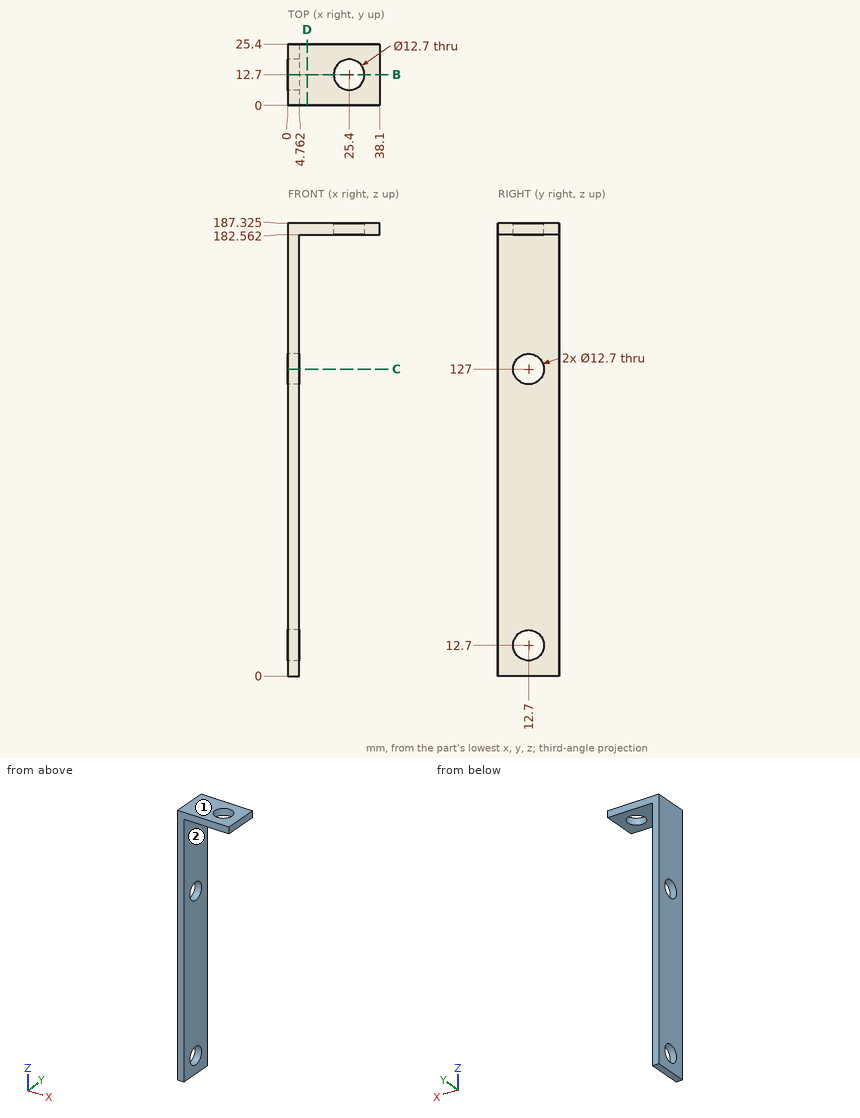
Source: three-view drawing plus pictorial views. Frame: mm from the lowest corner of the part. A direction names the side the tool comes from. Give positions to 0.01 mm unless a question says otherwise; leave off trailing zeros. Order: outer loops, then holes, each group sorted by start corner. A loop starts at its lowest first (then second) coordinate and runs counter-clockwise, first axis right, second up. Notation, with made-up numbers: (13, 35.25) -> (36, 35.25) arc R19 cw to (36, 63.25) -> close; hole circle Ø7 at (-20, 67.5). An arc over 180 degrees is marked (long way). Use a Markdown table: item, result.
Q1. Section C-C (z = 127). Return the cut outline in (x, y).
A:
| item | result |
|---|---|
| outline | (0, 0) -> (4.76, 0) -> (4.76, 6.35) -> (0, 6.35) -> close; (0, 19.05) -> (4.76, 19.05) -> (4.76, 25.4) -> (0, 25.4) -> close |
Q2. Material intervals for line 1 (Y direction, x = 25.4, z = 185.4); line 2 (X direction, y = 5, z = 92); line 3 (Z direction, x = 17, y = 13) (1 decimal), sorted ascending. Write a range as [from, to].
A:
| item | result |
|---|---|
| line 1 | [0, 6.35], [19.05, 25.4] |
| line 2 | [0, 4.76] |
| line 3 | [182.6, 187.3] |
Q3. Access query for the marked faces 1 and 2. Directions: +Z, -Z, +X, -X, +Y, -Y. A direction counts if a zero-diameter tool reaches every point of the face in a straight line with its end or side. Return the directions, or none.
A:
| item | result |
|---|---|
| face 1 | +Z, +X, -X, +Y, -Y |
| face 2 | -Z, +X, +Y, -Y |
Q4. Section B-B (y = 12.7). State how many separate pieces and enclosed holes the cut face has.
A:
| item | result |
|---|---|
| separate pieces | 4 |
| enclosed holes | 0 |
Q5. First-contact query: P1, Ø6, axis at x = 5.5, z = 166, coming from the -Y side; P2, Ø12.5, axis at x = 23, y = 14, coming from the -Z side; P3, Ø12, axis at y = 9, z = 102.5, coming from the +X side. Flat tips, straight axial feed; report the tip coordinate or a pass-through.
A:
| item | result |
|---|---|
| P1 | y = 0 |
| P2 | z = 182.56 |
| P3 | x = 4.76 |
Q6. Section D-D (x = 8). Return the cut outline in (y, z) (1 decimal).
A:
| item | result |
|---|---|
| outline | (0, 182.6) -> (25.4, 182.6) -> (25.4, 187.3) -> (0, 187.3) -> close |
